Geometry check sheet. Reference: the model listing, model coordinates, mm. Face numbers are marked on the shaded views. Coordinates: 2 decimals unless noted, no trailing zeros. Write each loop counter-clockwise with the first axis right and the second up, starting at its lowest first coordinate (ties: lowest second). Pieces come first, ordered by that corner, then holes. Notation, with made-up numbers: (-37, 43) - (2, 43) arc R18 ccw to (2, 52) - close; hole circle Ø2 at (-27, -1.5). An arc over 180 degrees is marked (long way). Answer as a JSON object with one key per item and string values. Group by question number.
from build123d import *

# Parameters (mm, degrees)
SKETCH1_R           = 25
BOSS_EXTRUDE1_DEPTH = 2
SKETCH2_R           = 5
BOSS_EXTRUDE2_DEPTH = 1.5
SKETCH3_R           = 3
BOSS_EXTRUDE3_DEPTH = 62.5
SKETCH4_R           = 1.05
CUT_EXTRUDE1_DEPTH  = 9


with BuildPart() as part:
    # Sketch1 → Boss-Extrude1 (new body)
    with BuildSketch(Plane(origin=(0, 0, 0), x_dir=(1, 0, 0), z_dir=(0, 1, 0))):
        with Locations(Location((0, 0, 0), (0, 0, 270))):
            Circle(SKETCH1_R)
    extrude(amount=BOSS_EXTRUDE1_DEPTH)

    # Sketch2 → Boss-Extrude2 (add)
    with BuildSketch(Plane(origin=(0, 2, 0), x_dir=(1, 0, 0), z_dir=(0, 1, 0))):
        with Locations(Location((0, 0, 0), (0, 0, 270))):
            Circle(SKETCH2_R)
    extrude(amount=BOSS_EXTRUDE2_DEPTH)

    # Sketch3 → Boss-Extrude3 (add)
    with BuildSketch(Plane(origin=(0, 3.5, 0), x_dir=(1, 0, 0), z_dir=(0, 1, 0))):
        with Locations(Location((0, 0, 0), (0, 0, 270))):
            Circle(SKETCH3_R)
    extrude(amount=BOSS_EXTRUDE3_DEPTH)

    # Sketch4 → Cut-Extrude1 (cut)
    with BuildSketch(Plane(origin=(0, 66, 0), x_dir=(1, 0, 0), z_dir=(0, 1, 0))):
        with Locations(Location((0, 0, 0), (0, 0, 270))):
            Circle(SKETCH4_R)
    extrude(amount=-CUT_EXTRUDE1_DEPTH, mode=Mode.SUBTRACT)

    # Mirror6: part across plane


with BuildPart() as part_1:
    add(part.part)
    add(part.part.mirror(Plane.ZX.offset(66)))


solid = part_1.part
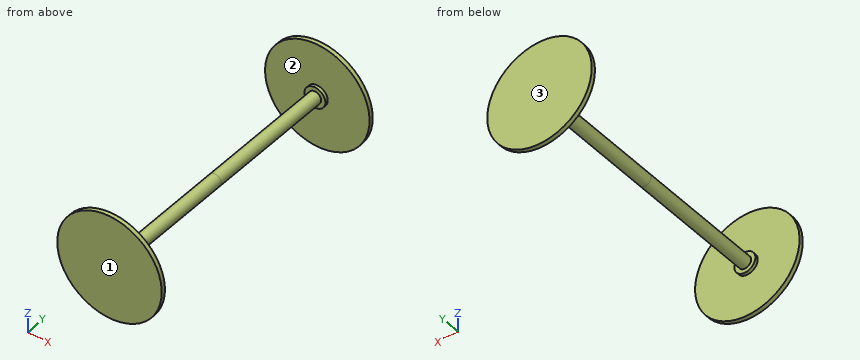
(1) Section check C-C (y = 50). Record the cut outline in (x, z).
(2) Material ranges on L1, parallel to Y at x = -11, z = -15.5; L2, parallel to X at y = 63, z = 0, recorded low to high. Write a range as [from, to].
(3) Gauge pin test, flat ends, axial feed: pin 1 (1 mm diameter, centred on y = 115.5, z = -2, fed in from +X); pin 2 (2.5 mm diameter, centred on x = 0, z = 0.5, fed in from -Y); pin 3 (12 mm diameter, centred on x = 12, y = 46.5, fed in from -Z); pin 4 (8 mm diameter, centred on y = 96, z = 4.5, fed in from -X). Record the tip position at first contact, or that the pin passes through.
(4) Draft check along Y on the marked faces 1, 2 and 3. Enter one of: +Y half, -Y half, draft (parallel to the pull), parting line (faces both ways), or undercut.
(5) Section check B-B (z = 18.5). Record the cut outline in (x, y), and give its area (3 significant figures).
(6) Section check A-A (x = 20). Record the cut outline in (y, z).
Conclusion:
{
 "1": {"outline": "circle Ø6 at (0, 0)"},
 "2": {"L1": "y = [0, 2], [130, 132]", "L2": "x = [-3, -1.05], [1.05, 3]"},
 "3": {"pin 1": "stops at x = 2.6", "pin 2": "stops at y = 0", "pin 3": "passes through", "pin 4": "stops at x = -2.96"},
 "4": {"face 1": "-Y half", "face 2": "undercut", "face 3": "+Y half"},
 "5": {"outline": "(-16.82, 0) - (16.82, 0) - (16.82, 2) - (-16.82, 2) - close; (-16.82, 130) - (16.82, 130) - (16.82, 132) - (-16.82, 132) - close", "area": "135 mm^2"},
 "6": {"outline": "(0, -15) - (2, -15) - (2, 15) - (0, 15) - close; (130, -15) - (132, -15) - (132, 15) - (130, 15) - close"}
}
